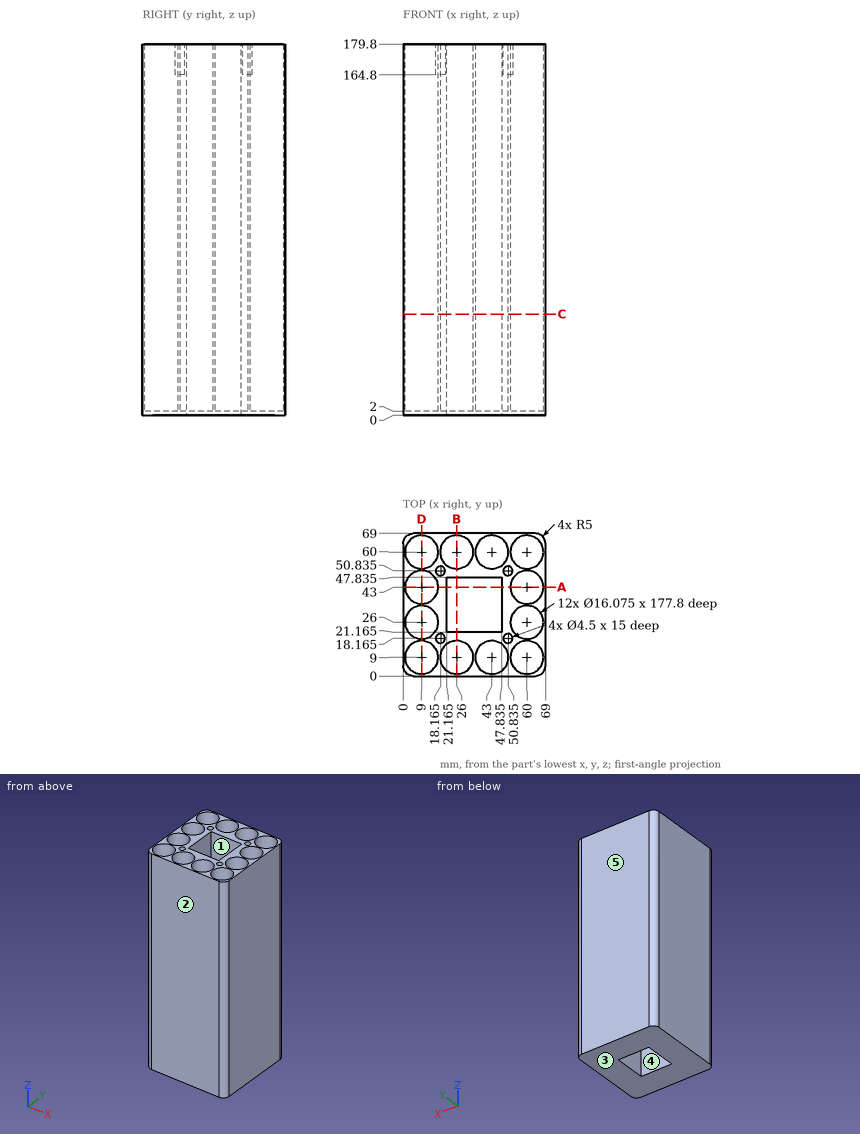
The figure shows three views and two pictorial views of one solid part (mm, origin at its lowest corner). Answer the questions. A direction names the side the tool comes from. Coordinates: 2 decimals unless noted, no trailing zeros. Loops run counter-clockwise (first coordinate to the right, second up) from the corner with the lowest first, then second, coordinate; pieces in that order, holes last. Notation, with made-up numbers: (20, 48) - (54, 48) arc R14 cw to (54, 73) - close; hole circle Ø11 at (43.25, 56). An arc over 180 degrees is marked (long way). Answer in a Markdown table with one row per item.
Q1. Find section D-D on x = 9. Write down the section's boundary in (y, z), plus the area to 3 significant figures.
Here are the results:
| item | result |
|---|---|
| outline | (0, 0) - (69, 0) - (69, 179.8) - (68.04, 179.8) - (68.04, 2) - (51.96, 2) - (51.96, 179.8) - (51.04, 179.8) - (51.04, 2) - (34.96, 2) - (34.96, 179.8) - (34.04, 179.8) - (34.04, 2) - (17.96, 2) - (17.96, 179.8) - (17.04, 179.8) - (17.04, 2) - (0.96, 2) - (0.96, 179.8) - (0, 179.8) - close |
| area | 974 mm^2 |
Q2. For the marked faces 1 and 2, determine the directions among +Z, -Z, +X, -X, +Y, -Y from which every point of the face is accessible in a straight line to the end or side of a thin tool.
Here are the results:
| item | result |
|---|---|
| face 1 | +Z, -Z |
| face 2 | +Z, -Z, +X, -X, -Y |
Q3. Find section A-A on y = 43. Write down the section's boundary in (x, z) (1 decimal).
Here are the results:
| item | result |
|---|---|
| outline | (0, 0) - (21.2, 0) - (21.2, 179.8) - (17, 179.8) - (17, 2) - (1, 2) - (1, 179.8) - (0, 179.8) - close; (47.8, 0) - (69, 0) - (69, 179.8) - (68, 179.8) - (68, 2) - (52, 2) - (52, 179.8) - (47.8, 179.8) - close |
Q4. The mould has two halves that part along Y. Classify the marked faces 3, 4 and 5: pulls with the +Y half, pulls with the -Y half, needs draft (parallel to the pull), parting line crosses it, or undercut.
Here are the results:
| item | result |
|---|---|
| face 3 | needs draft |
| face 4 | undercut |
| face 5 | pulls with the +Y half |
Q5. Given P1, Ø5, axis at x = 25.5, y = 64, coming from the +Z side; P2, Ø2, axis at x = 17.5, y = 50, coming from the +Z side, each flat-ended and moving along its own axis, determine where each tip first touches the part or whether it passes through.
Here are the results:
| item | result |
|---|---|
| P1 | stops at z = 2 |
| P2 | stops at z = 164.8 |
Q6. Straight lines are drawn through the part: line 1 along X through (y, z) = (6, 168); line 2 along X through (y, z) = (46.5, 70) (3 decimals); line 3 along X through (y, z) = (40, 26) (3 decimals). For each, find the intervals that lie inside material, in ascending order. Write a range as [from, to].
Here are the results:
| item | result |
|---|---|
| line 1 | x = [0, 1.54], [16.46, 18.54], [33.46, 35.54], [50.46, 52.54], [67.46, 69] |
| line 2 | x = [0, 1.765], [16.235, 21.165], [47.835, 52.765], [67.235, 69] |
| line 3 | x = [0, 1.543], [16.457, 21.165], [47.835, 52.543], [67.457, 69] |
Q7. Find section C-C on z = 49. Count the separate pieces of the cut face and the enclosed holes in it, plus the area to 3 significant figures.
Here are the results:
| item | result |
|---|---|
| separate pieces | 1 |
| enclosed holes | 13 |
| area | 1,590 mm^2 |
